from build123d import *

# Parameters (mm, degrees)
SKETCH1_W           = 70
SKETCH1_H           = 70
BOSS_EXTRUDE1_DEPTH = 3.175
SKETCH2_W           = 1
SKETCH2_H           = 16.56370183
CUT_EXTRUDE1_DEPTH  = 3.175
SKETCH3_W           = 40
SKETCH3_H           = 20.7
CUT_EXTRUDE2_DEPTH  = 3.175


with BuildPart() as part:
    # Sketch1 → Boss-Extrude1 (new body)
    with BuildSketch(Plane(origin=(0, 0, 0), x_dir=(1, 0, 0), z_dir=(0, 1, 0))):
        Rectangle(SKETCH1_W, SKETCH1_H)
    extrude(amount=BOSS_EXTRUDE1_DEPTH)

    # Sketch2 → Cut-Extrude1 (cut)
    with BuildSketch(Plane(origin=(0, 3.175, 0), x_dir=(1, 0, 0), z_dir=(0, 1, 0))):
        with Locations((0.5, 26.718149085)):
            Rectangle(SKETCH2_W, SKETCH2_H)
    extrude(amount=-CUT_EXTRUDE1_DEPTH, mode=Mode.SUBTRACT)

    # Sketch3 → Cut-Extrude2 (cut)
    with BuildSketch(Plane(origin=(0, 0, 0), x_dir=(-1, 0, 0), z_dir=(0, -1, 0))):
        with Locations((0.662640496, -11.168119056)):
            Rectangle(SKETCH3_W, SKETCH3_H)
    extrude(amount=-CUT_EXTRUDE2_DEPTH, mode=Mode.SUBTRACT)


solid = part.part
Model file for the job. Use its own axes, mm. A direction names the side the tool comes from. Coordinates: 2 decimals unless noted, no trailing zeros. Write each loop counter-clockwise with the first axis right and the second up, starting at its lowest first coordinate (ties: lowest second). Pieces come first, ordered by that corner, then holes. Notation, with made-up numbers: (81.25, -24) -> (87.25, -24) arc R24 ccw to (87.25, 5) -> close; hole circle Ø10 at (-9.75, 85). An arc over 180 degrees is marked (long way). One line per item, written item: value. Start each with the question number.
1) Probe probe 1 along Z at (x, y) = (7.5, 1.5); probe 2 along X at (y, z) = (1.25, 12); probe 3 along X at (y, z) = (0.3, -22). List the from-to ranges inside material, lowest first.
2) Slice it at A-A on x = -4.5. Write the cut outline in (y, z) (3 decimals), then the cut area to 3 significant figures.
3) Slice it at B-B on z = 4. Write the cut outline in (x, y) (3 decimals).
4) Flat gauge pin, fed straight in: pin 1 Ø0.5 at (x, y) = (0.5, 2) entering from -Z. Where does the tip first touch, or does it go through?
5) Slice it at C-C on y = 1.35. Write the cut outline in (x, z).
6) Pull direction Z, two halves, no side cores. Call faces 1 (the face through (-18, 2, -35)), 2 (the face through (0, 0, 0)), 3 (the face through (-20.663, 2, 11)): +Z half, -Z half, draft (parallel to the pull), parting line (faces both ways), or undercut.
7) Which spindle directions (+Z, -Z, +X, -X, +Y, -Y) get a long thin tool onto all of the face, cutting with end or side? Do faces 4 (the face through (0, 2, -27)), 5 (the face through (0, 2, 35)), 6 (the face through (19.337, 2, 11)). Say none if no direction does.
Answers follow:
1. probe 1: -35 to 0.82, 21.52 to 35
1. probe 2: -35 to -20.66, 19.34 to 35
1. probe 3: -35 to 0, 1 to 35
2. outline: (0, -35) -> (3.175, -35) -> (3.175, 0.818) -> (0, 0.818) -> close; (0, 21.518) -> (3.175, 21.518) -> (3.175, 35) -> (0, 35) -> close
2. area: 157 mm2
3. outline: (-35, 0) -> (-20.663, 0) -> (-20.663, 3.175) -> (-35, 3.175) -> close; (19.337, 0) -> (35, 0) -> (35, 3.175) -> (19.337, 3.175) -> close
4. pin 1: z = -18.44
5. outline: (-35, -35) -> (0, -35) -> (0, -18.44) -> (1, -18.44) -> (1, -35) -> (35, -35) -> (35, 35) -> (-35, 35) -> close; hole (-20.66, 0.82) -> (19.34, 0.82) -> (19.34, 21.52) -> (-20.66, 21.52) -> close
6. face 1: -Z half
6. face 2: draft
6. face 3: undercut
7. face 4: -Z, +Y, -Y
7. face 5: +Z, +X, -X, +Y, -Y
7. face 6: +Y, -Y
